from build123d import *

# Parameters (mm, degrees)
SKETCH16_W           = 2.4
SKETCH16_H           = 4
BOSS_EXTRUDE11_DEPTH = 2.5
SKETCH19_R           = 1.25
CUT_EXTRUDE12_DEPTH  = 5
CUT_EXTRUDE13_DEPTH  = 10


with BuildPart() as part:
    # Sketch16 → Revolve1 (revolve)
    with BuildSketch(Plane(origin=(0, 0, 0), x_dir=(1, 0, 0), z_dir=(0, 1, 0))):
        with Locations((-1.2, -2)):
            Rectangle(SKETCH16_W, SKETCH16_H)
    revolve(axis=Axis((0, 0, -4.094545455), (0, 0, 1)))

    # Sketch18 → Boss-Extrude11 (add, symmetric)
    with BuildSketch(Plane(origin=(0, 0, 0), x_dir=(1, 0, 0), z_dir=(0, 1, 0))):
        with BuildLine():
            Line((0, -4), (-3.019312417, -4))
            ThreePointArc((-3.019312417, -4), (-3.287962221, -4.078304277), (-3.472466311, -4.288690869))
            Line((-3.472466311, -4.288690869), (-5.459461681, -8.549816191))
            ThreePointArc((-5.459461681, -8.549816191), (-5.564444011, -8.859084162), (-5.6, -9.183743583))
            Line((-5.6, -9.183743583), (-5.6, -13.084062043))
            ThreePointArc((-5.6, -13.084062043), (-4.674025149, -14.469881342), (-3.039339828, -14.144722215))
            Line((-3.039339828, -14.144722215), (4.843681451, -6.261700936))
            ThreePointArc((4.843681451, -6.261700936), (4.916904756, -6.08492424), (4.843681451, -5.908147545))
            Line((4.843681451, -5.908147545), (4.242640687, -5.307106781))
            Line((4.242640687, -5.307106781), (3.535533906, -6.014213562))
            Line((3.535533906, -6.014213562), (3.712310601, -6.190990258))
            ThreePointArc((3.712310601, -6.190990258), (3.785533906, -6.367766953), (3.712310601, -6.544543648))
            Line((3.712310601, -6.544543648), (-3.292893219, -13.549747468))
            ThreePointArc((-3.292893219, -13.549747468), (-4.382683432, -13.76652022), (-5, -12.842640687))
            Line((-5, -12.842640687), (-5, -9.316760381))
            ThreePointArc((-5, -9.316760381), (-4.964444011, -8.99210096), (-4.859461681, -8.682832988))
            Line((-4.859461681, -8.682832988), (-3.359461681, -5.466072607))
            ThreePointArc((-3.359461681, -5.466072607), (-2.805949413, -4.834912831), (-2, -4.6))
            Line((-2, -4.6), (0, -4.6))
            Line((0, -4.6), (2.017766953, -4.6))
            ThreePointArc((2.017766953, -4.6), (2.113437811, -4.619030117), (2.194543648, -4.673223305))
            Line((2.194543648, -4.673223305), (3.181980515, -5.660660172))
            Line((3.181980515, -5.660660172), (3.889087297, -4.953553391))
            Line((3.889087297, -4.953553391), (3.008757211, -4.073223305))
            ThreePointArc((3.008757211, -4.073223305), (2.927651373, -4.019030117), (2.831980515, -4))
            Line((2.831980515, -4), (0, -4))
        make_face()
    extrude(amount=BOSS_EXTRUDE11_DEPTH, both=True)

    # Sketch19 → Cut-Extrude12 (cut)
    with BuildSketch(Plane(origin=(0, 0, 0), x_dir=(-1, 0, 0), z_dir=(0, 0, -1))):
        Circle(SKETCH19_R)
    extrude(amount=-CUT_EXTRUDE12_DEPTH, mode=Mode.SUBTRACT)

    # Sketch22 → Revolve2 (revolve)
    with BuildSketch(Plane.XZ):
        with BuildLine():
            Line((0.424264069, 10.681118318), (-3.619403821, 14.724786208))
            ThreePointArc((-3.619403821, 14.724786208), (0.300410275, 15.99900138), (4.065863992, 14.322718241))
            Line((4.065863992, 14.322718241), (0.424264069, 10.681118318))
        make_face()
    revolve(axis=Axis((0, 0, 10.256854249), (0.7071067811865477, 0, 0.7071067811865474)))

    # Sketch23 → Cut-Extrude13 (cut)
    with BuildSketch(Plane(origin=(5.552691193, 0, 5.552691193), x_dir=(-0.7071067811865476, 0, 0.7071067811865476), z_dir=(-0.7071067811865476, 0, -0.7071067811865476))):
        with BuildLine():
            Line((11.339560411, 4), (3.165821976, 4))
            ThreePointArc((3.165821976, 4), (7.252691193, 5.718609971), (11.339560411, 4))
        make_face()
        with BuildLine():
            Line((11.339560411, -4), (3.165821976, -4))
            ThreePointArc((3.165821976, -4), (7.252691193, -5.718609971), (11.339560411, -4))
        make_face()
    extrude(amount=-CUT_EXTRUDE13_DEPTH, mode=Mode.SUBTRACT)


solid = part.part
Work out the finished part from the listing and answer in its coordinate system (mm). A direction names the side the tool comes from. Give positions to 0.01 mm unless a question says otherwise; leave off trailing zeros. Loops run counter-clockwise (first coordinate to the right, second up) from the corner with the lowest first, then second, coordinate; pieces in that order, holes last. Notation, with made-up numbers: M 81,9 L 101,9 A16 cw 101,17 Z; hole C 43,4 d11. An arc over 180 degrees is marked long. Use CSV: the item, a comma, the result in double quotes.
1) Find section C-C on z = 1.5. Write down the section's boundary in (x, y), plus the area to 3 significant figures.
Answer:
outline,"C 0,0 d4.8; hole C 0,0 d2.5"
area,"13.2 mm^2"
2) Which of the six approach directions +Z, -Z, +X, -X, +Y, -Y give full straight-line access (tool end or side, diameter ignored) to faces 4 (the cylindrical face through (0.27, -1.22, 2.27)), 5 (the flat face through (0.4, 2.5, 10.1)), 6 (the flat face through (0.167, -2.723, 10.938)), 7 (the flat face through (-5, 0, 11))?
Answer:
face 4,"-Z"
face 5,"-Z, -X, +Y"
face 6,"none"
face 7,"+Y, -Y"
3) Determine the mould class of faces 1 (the flat face through (-4.12, 0.04, 7.1)), 2 (the flat face through (-5.6, 0, 11)), 3 (the flat face through (0.4, -2.5, 10.1)) for opening direction X: released by +X, released by -X, zero draft, split by the parting line, or undercut.
Answer:
face 1,"undercut"
face 2,"released by -X"
face 3,"zero draft"
4) Consider L1, parallel to Y at x = 0, z = 2.25; L2, parallel to Y at x = -2.75, z = 4.75; L3, parallel to X at y = -0.5, z = 12.5. Determine where each line is inside the solid, lowest interval first.
Answer:
L1,"-2.4 to -1.25, 1.25 to 2.4"
L2,"-2.5 to 2.5"
L3,"-5.6 to -5, -2.24 to 5.27"
5) Find section A-A on z = 12.5. Write down the section's boundary in (x, y).
Answer:
outline,"M -5.6,-2.5 L -5,-2.5 L -5,2.5 L -5.6,2.5 Z; M -2.24,-2.5 L -1.39,-2.5 L -1.39,-4 L 3.47,-4 A5.29 ccw 3.47,4 L -1.39,4 L -1.39,2.5 L -2.24,2.5 Z"
6) Given P1, Ø5.5, axis at x = -0.5, z = 10.5, coming from the -Y side; P2, Ø2, axis at x = -0.5, y = 1, coming from the +Z side; P3, Ø2, axis at x = 0, y = 0, coming from the -Z side; P4, Ø2, axis at x = -1, y = -2.5, coming from the +Z side, each flat-ended and moving along its own axis, determine where each tip first touches the part or whether it passes through.
Answer:
P1,"y = -4"
P2,"z = 16.01"
P3,"z = 9.26"
P4,"z = 15.75"
7) Find section B-B on x = -0.25. Write down the section's boundary in (y, z).
Answer:
outline,"M -4,11.36 L -2.5,11.36 L -2.5,10.51 L 2.5,10.51 L 2.5,11.36 L 4,11.36 L 4,14.38 A5.74 ccw -4,14.38 Z; M -2.5,4 L -2.39,4 L -2.39,0 L -1.22,0 L -1.22,4.6 L -2.5,4.6 Z; M 1.22,0 L 2.39,0 L 2.39,4 L 2.5,4 L 2.5,4.6 L 1.22,4.6 Z"
